The listing builds one solid part. Answer for the finished solid, in the listing's coordinates (mm). A direction names the side the tool comes from. Give positions to 0.01 mm unless a question says otherwise; leave off trailing zeros. Write each loop counter-clockwise with the first axis right and the second up, starting at its lowest first coordinate (ties: lowest second). Pieces come first, ordered by that corner, then holes. Notation, with made-up numbers: (-22.75, -9.5) - (21.25, -9.5) arc R20 ccw to (21.25, 21.5) - close; hole circle Ø6 at (-5.5, 89.25). An arc over 180 degrees is marked (long way). Use a Markdown table: item, result. Add a question column.
from build123d import *

# Parameters (mm, degrees)
SKETCH1_W          = 25
SKETCH1_H          = 15
SKETCH2_R          = 3.9
SKETCH2_R_2        = 1.45
CUT_EXTRUDE1_DEPTH = 53
SKETCH3_R          = 1.5
CUT_EXTRUDE2_DEPTH = 53


with BuildPart() as part:
    # Sketch1 → Revolve1 (revolve)
    with BuildSketch(Plane(origin=(0, 0, 0), x_dir=(0, 0, -1), z_dir=(1, 0, 0))):
        Polygon((0, 20), (0, 15), (25, 15), (35, 15), (35, 20), align=None)
        with Locations((12.5, 7.5)):
            Rectangle(SKETCH1_W, SKETCH1_H)
        Polygon((25, 0), (0, 0), (0, -5), (35, -5), (35, 0), align=None)
    revolve(axis=Axis((0, 0, 0), (0, 1, 0)))

    # Sketch2 → Cut-Extrude1 (cut)
    with BuildSketch(Plane(origin=(0, 20, 0), x_dir=(1, 0, 0), z_dir=(0, 1, 0))):
        with Locations(Location((0, 0, 0), (0, 0, 270))):
            Circle(SKETCH2_R)
        with Locations(Location((0, 12, 0), (0, 0, 270))):
            Circle(SKETCH2_R_2)
        with Locations(Location((12, 0, 0), (0, 0, 270))):
            Circle(SKETCH2_R_2)
        with Locations(Location((0, -12, 0), (0, 0, 270))):
            Circle(SKETCH2_R_2)
        with Locations(Location((-12, 0, 0), (0, 0, 270))):
            Circle(SKETCH2_R_2)
    extrude(amount=-CUT_EXTRUDE1_DEPTH, mode=Mode.SUBTRACT)

    # Sketch3 → Cut-Extrude2 (cut)
    with BuildSketch(Plane(origin=(0, 20, 0), x_dir=(1, 0, 0), z_dir=(0, 1, 0))):
        with Locations(Location((0, 30, 0), (0, 0, 90))):
            Circle(SKETCH3_R)
    extrude(amount=-CUT_EXTRUDE2_DEPTH, mode=Mode.SUBTRACT)


solid = part.part
1. The part is cut by section B-B (z = 0). Give the vertices of the cut face in (x, y), and give its area (3 significant figures).
2. Which of the six approach directions +Z, -Z, +X, -X, +Y, -Y give full straight-line access (tool end or side, diameter ignored) to faces 1 (the flat face through (-23, 0, 11)), 2 (the flat face through (7, 20, 0))?
3. For a pull along X with two mould halves and no side action, classify faces 3 (the flat face through (-8, 15, -24)), 4 (the cylindrical face through (-7.509, 7.605, -23.846)), 5 (the cylindrical face through (10.584, 7.675, -0.314)) as released by +X, released by -X, zero draft, split by the parting line, or undercut.
4. Consider L1, parallel to X at y = 13.75, z = 0; L2, parallel to Y at x = 30.5, z = -1; L3, parallel to X at y = -1, z = -0.5. Determine where each line is inside the solid, lowest interval first. Write a range as [from, to].
5. The part is cut by section A-A (x = -28). Give the vertices of the cut face in (y, z).
6. The part is cut by section D-D (x = 0). Count the separate pieces of the cut face and the enclosed holes in it, and give its area (3 significant figures).
7. The part is cut by section C-C (y = 16.5). Give the vertices of the cut face in (x, z), and give its area (3 significant figures).
8. Given P1, Ø2, axis at x = 13.5, y = 7, coming from the -Z side; P2, Ø3.5, axis at x = 12, z = 0, coming from the +Y side; P3, Ø2, axis at x = 10.5, y = 0.5, coming from the +Z side; P4, Ø8, axis at x = -0.5, y = 7.5, coming from the +Z side, each flat-ended and moving along its own axis, determine where each tip first touches the part or whether it passes through.
Check values:
| question | item | result |
|---|---|---|
| 1 | outline | (-35, -5) - (-13.45, -5) - (-13.45, 20) - (-35, 20) - (-35, 15) - (-25, 15) - (-25, 0) - (-35, 0) - close; (-10.55, -5) - (-3.9, -5) - (-3.9, 20) - (-10.55, 20) - close; (3.9, -5) - (10.55, -5) - (10.55, 20) - (3.9, 20) - close; (13.45, -5) - (35, -5) - (35, 0) - (25, 0) - (25, 15) - (35, 15) - (35, 20) - (13.45, 20) - close |
| 1 | area | 1,110 mm2 |
| 2 | face 1 | none |
| 2 | face 2 | +Z, -Z, +X, -X, +Y |
| 3 | face 3 | zero draft |
| 3 | face 4 | split by the parting line |
| 3 | face 5 | undercut |
| 4 | L1 | x = [-25, -13.45], [-10.55, -3.9], [3.9, 10.55], [13.45, 25] |
| 4 | L2 | y = [-5, 0], [15, 20] |
| 4 | L3 | x = [-35, -13.36], [-10.64, -3.87], [3.87, 10.64], [13.36, 35] |
| 5 | outline | (-5, -21) - (0, -21) - (0, 21) - (-5, 21) - close; (15, -21) - (20, -21) - (20, 21) - (15, 21) - close |
| 6 | separate pieces | 6 |
| 6 | enclosed holes | 0 |
| 6 | area | 1,080 mm2 |
| 7 | outline | circle Ø70 at (0, 0); hole circle Ø2.9 at (-12, 0); hole circle Ø7.8 at (0, 0); hole circle Ø3 at (0, -30); hole circle Ø2.9 at (0, -12); hole circle Ø2.9 at (0, 12); hole circle Ø2.9 at (12, 0) |
| 7 | area | 3,770 mm2 |
| 8 | P1 | stops at z = -21.65 |
| 8 | P2 | stops at y = 20 |
| 8 | P3 | stops at z = 33.65 |
| 8 | P4 | stops at z = 25 |
